The model under review builds one solid part; all positions refer to its coordinate system, in mm. Give positions to 0.01 mm unless a question says otherwise; leave off trailing zeros. Loops run counter-clockwise (first coordinate to the right, second up) from the corner with the lowest first, then second, coordinate; pieces in that order, holes last. Notation, with made-up numbers: M 41.5,45 L 63.5,45 A13 cw 63.5,70 Z; hole C 32,-24.5 d6. An arc over 180 degrees is marked long. Put each result on its own line as item: value. Start each with the question number.
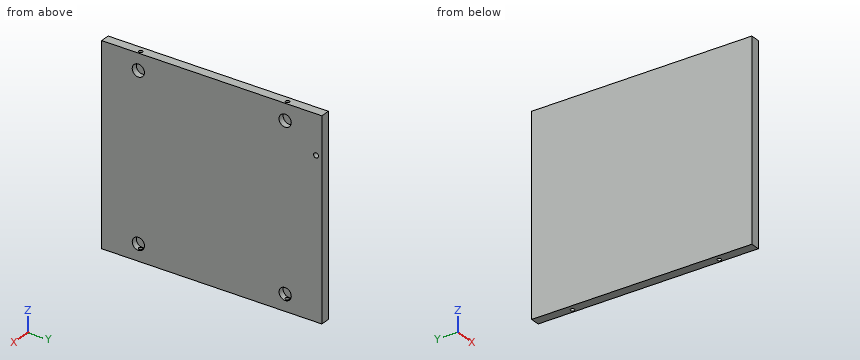
```python
from build123d import *

# Parameters (mm, degrees)
F0_W     = 450
F0_H     = 400
F1_DEPTH = 19
F2_R     = 12.5
F3_DEPTH = 12
F5_D     = 8
F5_DEPTH = 22
F5_TIP   = 2.4034424761
F7_D     = 10
F7_DEPTH = 13
F7_TIP   = 3.0043030951


# Not quite as in the source:
# - a pattern or mirror of a feature is missing from the dataset's text; its kind, count and spacing are read off the source's solid


with BuildPart() as f1:
    # F0 (on Right) → F1 (new body)
    with BuildSketch(Plane.YZ):
        Rectangle(F0_W, F0_H)
    extrude(amount=-F1_DEPTH)

    # F2 (on face) → F3 (cut)
    with BuildSketch(Plane.YZ):
        with Locations((-150, -166.5)):
            Circle(F2_R)
        with Locations((150, -166.5)):
            Circle(F2_R)
        with Locations((-150, 166.5)):
            Circle(F2_R)
        with Locations((150, 166.5)):
            Circle(F2_R)
    extrude(amount=-F3_DEPTH, mode=Mode.SUBTRACT)

    # F5
    with Locations(Plane.XY.offset(200)):
        with Locations((-7, 150), (-7, -150)):
            f5 = Hole(F5_D / 2, depth=F5_DEPTH)
            with Locations((0, 0, -(F5_DEPTH + F5_TIP / 2))):  # 118° drill point
                Cone(0, F5_D / 2, F5_TIP, mode=Mode.SUBTRACT)

    # F5_copies: F5 across plane
    add(f5.mirror(Plane(origin=(0, 0, 2.1e-05), x_dir=(-1, 0, 0), z_dir=(0, 0, -1))), mode=Mode.SUBTRACT)

    # F7
    with Locations(Plane.YZ):
        with Locations((213, 120)):
            Hole(F7_D / 2, depth=F7_DEPTH)
            with Locations((0, 0, -(F7_DEPTH + F7_TIP / 2))):  # 118° drill point
                Cone(0, F7_D / 2, F7_TIP, mode=Mode.SUBTRACT)


solid = f1.part
```
Item 1: Consider section A-A, the plane x = -7. Write out the cut boundary in (y, z).
Item 2: To check wall thickness, follow L1, parallel to Y at x = -7, z = 195.25; L2, parallel to X at y = 150, z = 185; L3, parallel to Y at x = -6.25, z = 120. State the ranges of each line that lie inside material, in increasing order. Write a range as [from, to].
Item 3: Clearance check with flat-ended pins moving along their axes: pin 1 Ø12.5 at (y, z) = (-154.5, 169) entering from +X; pin 2 Ø5 at (x, y) = (-7, -150) entering from +Z. State where each tip first meets the part, or that it passes through.
Item 4: Consider section B-B, the plane z = -166.5. Write out the cut boundary in (x, y), plus the area to 3 significant figures.
Report:
1. outline: M -225,-200 L -154,-200 L -154,-178.34 A12.5 cw long -146,-178.34 L -146,-200 L 146,-200 L 146,-178.34 A12.5 cw long 154,-178.34 L 154,-200 L 225,-200 L 225,200 L 154,200 L 154,178.34 A12.5 cw long 146,178.34 L 146,200 L -146,200 L -146,178.34 A12.5 cw long -154,178.34 L -154,200 L -225,200 Z; hole C 213,120 d10
2. L1: [-225, -154], [-146, 146], [154, 225]
2. L2: [-19, -11], [-3, 0]
2. L3: [-225, 208], [218, 225]
3. pin 1: x = -12
3. pin 2: z = 154.25
4. outline: M -19,-225 L 0,-225 L 0,-162.5 L -12,-162.5 L -12,-137.5 L 0,-137.5 L 0,137.5 L -12,137.5 L -12,162.5 L 0,162.5 L 0,225 L -19,225 Z
4. area: 7,950 mm²
